CAD build for the part. Positions are in the model's coordinates, mm. A direction names the side the tool comes from. Give positions to 0.01 mm unless a question says otherwise; leave off trailing zeros. Order: outer loops, then holes, each group sorted by start corner. A loop starts at its lowest first (then second) coordinate and runs counter-clockwise, first axis right, second up. Notation, with made-up numbers: M 21.25,42.5 L 51.25,42.5 A17 ccw 51.25,75.5 Z; hole C 21.25,-15.5 d4. An arc over 180 degrees is marked long. Put each result on its own line as item: value. Start each with the question number.
1) Tool access for faces 4 (the face through (27, -4, 3)), 5 (the face through (26.15, -9.94, 2.46)): list every direction of +Z, -Z, +X, -X, +Y, -Y with a clear straight run to the whole face (end or side of a thin tool).
2) Drill centre lines: line 1 (Y direction, x = 0, z = 1.95); line 2 (X direction, y = -0.75, z = 3.3); line 3 (Y direction, x = 23, z = 3.8). Where is each one in solid material? Low to high. Write a range as [from, to].
3) Pin check, flat tips, straight feed: pin 1 (1 mm diameter, centred on x = 34.5, y = -5, fed in from -Z); pin 2 (1.9 mm diameter, centred on x = -7, y = 0, fed in from -Z); pin 3 (2.5 mm diameter, centred on x = 26.5, z = 1.5, fed in from +Y); pin 4 (1 mm diameter, centred on y = -8.5, z = 3.5, fed in from -X). Stop position of each tip, or through.
4) Two-plate mould, pull along Y, no slides. Class faces 1 (the face through (23, -5, 0)), 2 (the face through (25.452, 9.996, 2.465)), 3 (the face through (4.896, -2.03, 2.465)): released by +Y, released by -Y, zero draft, split by the parting line, or undercut.
5) Cut at D-D (y = 7). Write the cut outline in (x, z).
6) Cut at A-A (y = 0). Write the cut outline in (x, z).
7) Cut at B-B (x = 50). Write the cut outline in (y, z).
8) Cut at C-C (z = 4.3). Write the cut outline in (x, y).
```python
from build123d import *

# Parameters (mm, degrees)
SKETCH_1_R          = 5.3
SKETCH_1_R_2        = 3.05
SKETCH_1_R_3        = 1.55
EXTRUDE_1_DEPTH     = 5
CUT_EXTRUDE_1_DEPTH = 10


with BuildPart() as part:
    # 草图1 → 凸台-拉伸1 (new body)
    with BuildSketch(Plane.XY):
        with BuildLine():
            Line((0.96, 11.961538363), (50.64, 7.974358908))
            ThreePointArc((50.64, 7.974358908), (58, 0), (50.64, -7.974358908))
            Line((50.64, -7.974358908), (0.96, -11.961538363))
            ThreePointArc((0.96, -11.961538363), (-12, 0), (0.96, 11.961538363))
        make_face()
        Circle(SKETCH_1_R, mode=Mode.SUBTRACT)
        with Locations((50, 0)):
            Circle(SKETCH_1_R_2, mode=Mode.SUBTRACT)
        with Locations((-7, 0)):
            Circle(SKETCH_1_R_3, mode=Mode.SUBTRACT)
        with Locations((7, 0)):
            Circle(SKETCH_1_R_3, mode=Mode.SUBTRACT)
        with Locations((0, 7)):
            Circle(SKETCH_1_R_3, mode=Mode.SUBTRACT)
        with Locations((0, -7)):
            Circle(SKETCH_1_R_3, mode=Mode.SUBTRACT)
    extrude(amount=EXTRUDE_1_DEPTH)

    # 草图2 → 切除-拉伸1 (cut)
    with BuildSketch(Plane.XY.offset(5)):
        with BuildLine():
            Line((15, 4), (39, 4))
            ThreePointArc((39, 4), (43, 0), (39, -4))
            Line((39, -4), (15, -4))
            ThreePointArc((15, -4), (11, 0), (15, 4))
        make_face()
    extrude(amount=-CUT_EXTRUDE_1_DEPTH, mode=Mode.SUBTRACT)


solid = part.part
```
Solution:
1. face 4: +Z, -Z
1. face 5: +Z, -Z, +X, -Y
2. line 1: [-12, -8.55], [-5.45, -5.3], [5.3, 5.45], [8.55, 12]
2. line 2: [-11.98, -8.36], [-5.64, -5.25], [5.25, 5.64], [8.36, 11.07], [42.93, 47.04], [52.96, 57.96]
2. line 3: [-10.19, -4], [4, 10.19]
3. pin 1: z = 0
3. pin 2: through
3. pin 3: y = 10.01
3. pin 4: x = -8.94
4. face 1: zero draft
4. face 2: released by +Y
4. face 3: undercut
5. outline: M -9.75,0 L -1.55,0 L -1.55,5 L -9.75,5 Z; M 1.55,0 L 53.87,0 L 53.87,5 L 1.55,5 Z
6. outline: M -12,0 L -8.55,0 L -8.55,5 L -12,5 Z; M -5.45,0 L -5.3,0 L -5.3,5 L -5.45,5 Z; M 5.3,0 L 5.45,0 L 5.45,5 L 5.3,5 Z; M 8.55,0 L 11,0 L 11,5 L 8.55,5 Z; M 43,0 L 46.95,0 L 46.95,5 L 43,5 Z; M 53.05,0 L 58,0 L 58,5 L 53.05,5 Z
7. outline: M -8.03,0 L -3.05,0 L -3.05,5 L -8.03,5 Z; M 3.05,0 L 8.03,0 L 8.03,5 L 3.05,5 Z
8. outline: M 0.96,-11.96 L 50.64,-7.97 A8 ccw 50.64,7.97 L 0.96,11.96 A12 ccw long Z; hole C -7,0 d3.1; hole C 0,0 d10.6; hole C 0,-7 d3.1; hole C 0,7 d3.1; hole C 7,0 d3.1; hole M 15,-4 L 39,-4 A4 ccw 39,4 L 15,4 A4 ccw Z; hole C 50,0 d6.1
